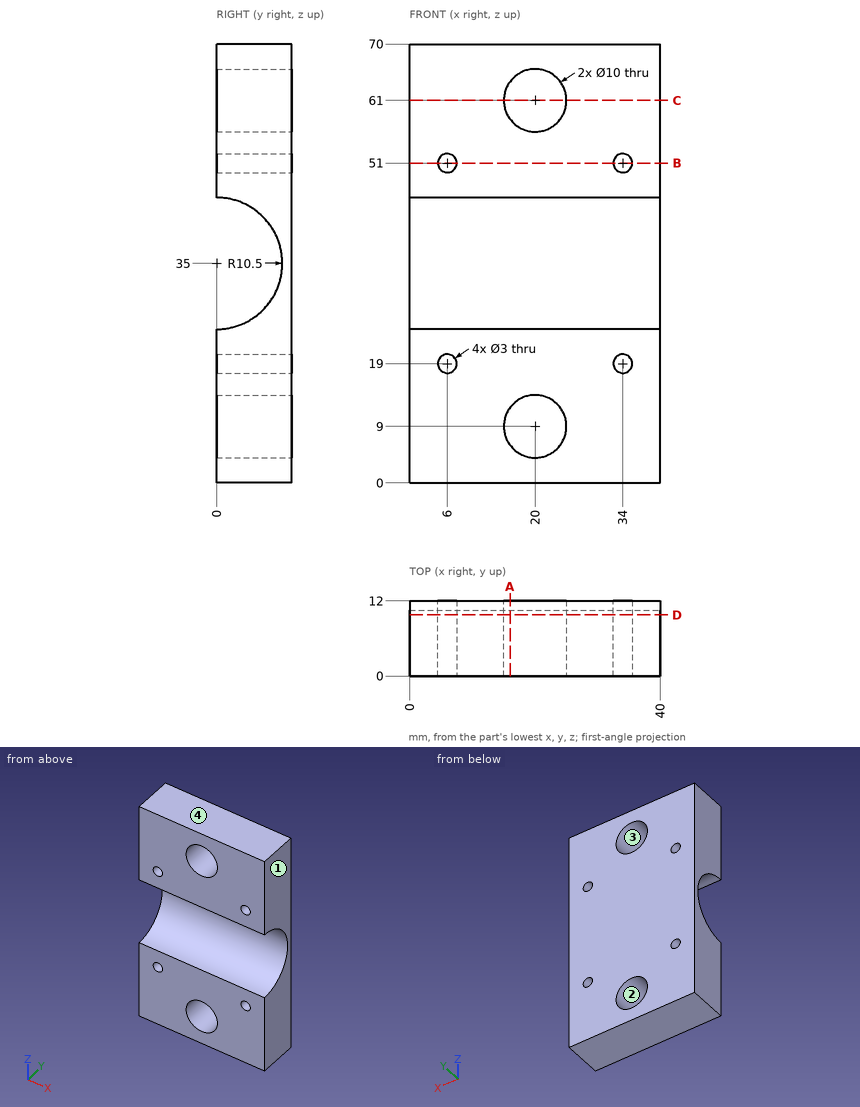
For this review, use the dimensioned drawing (mm, ordinates from the lowest corner) and the shaded views. Round coordinates to 2 decimals unless told otherwise and drop trailing zeros. Write each loop counter-clockwise with the first axis right and the second up, starting at its lowest first coordinate (ties: lowest second). Pieces come first, ordered by that corner, then holes. Notation, with made-up numbers: (-5.75, 60.25) -> (7.25, 60.25) arc R8 ccw to (7.25, 68.25) -> close; hole circle Ø1 at (11.25, 38). An arc over 180 degrees is marked (long way). One line per item, written item: value. Start each with the question number.
Q1. Add section C-C (z = 61). Give the boundary of the cut face in (x, y), then the cut area to 3 significant figures.
Q2. Add section A-A (x = 16). Give the boundary of the cut face in (y, z).
Q3. To check wall thickness, follow probe 1 along Z at (x, y) = (20, 4.5); probe 2 along Z at (x, y) = (20, 4.25); probe 3 along Z at (x, y) = (12, 7.75). State the ranges of each line that lie inside material, in increasing order.
Q4. Add section B-B (z = 51). Give the boundary of the cut face in (x, y), then the cut area to 3 significant figures.
Q5. Add section D-D (y = 9.75). Give the boundary of the cut face in (x, z), then the cut area to 3 significant figures.
Q6. The part is to be moulded in two halves that separate along X. For the marked faces 1, 2, 3 and 4, say which applies: pulls with the +X half, pulls with the -X half, needs draft (parallel to the pull), parting line crosses it, or undercut.
Q7. Insertion check: P1, Ø6, axis at x = 20, z = 9, coming from the -Y side. The pin has a flat end and moves straight along its axis. Give the tip position at first contact, or say it passes through.
Response:
1. outline: (0, 0) -> (15, 0) -> (15, 12) -> (0, 12) -> close; (25, 0) -> (40, 0) -> (40, 12) -> (25, 12) -> close
1. area: 360 mm^2
2. outline: (0, 0) -> (12, 0) -> (12, 6) -> (0, 6) -> close; (0, 12) -> (12, 12) -> (12, 58) -> (0, 58) -> (0, 45.5) arc R10.5 cw to (0, 24.5) -> close; (0, 64) -> (12, 64) -> (12, 70) -> (0, 70) -> close
3. probe 1: z = 0 to 4, 14 to 25.51, 44.49 to 56, 66 to 70
3. probe 2: z = 0 to 4, 14 to 25.4, 44.6 to 56, 66 to 70
3. probe 3: z = 0 to 27.92, 42.08 to 70
4. outline: (0, 0) -> (4.5, 0) -> (4.5, 12) -> (0, 12) -> close; (7.5, 0) -> (32.5, 0) -> (32.5, 12) -> (7.5, 12) -> close; (35.5, 0) -> (40, 0) -> (40, 12) -> (35.5, 12) -> close
4. area: 408 mm^2
5. outline: (0, 0) -> (40, 0) -> (40, 31.1) -> (0, 31.1) -> close; (0, 38.9) -> (40, 38.9) -> (40, 70) -> (0, 70) -> close; hole circle Ø3 at (6, 19); hole circle Ø3 at (6, 51); hole circle Ø10 at (20, 9); hole circle Ø10 at (20, 61); hole circle Ø3 at (34, 19); hole circle Ø3 at (34, 51)
5. area: 2,300 mm^2
6. face 1: pulls with the +X half
6. face 2: undercut
6. face 3: undercut
6. face 4: needs draft
7. P1: passes through
